Autodesk Inventor part; units mm, degrees
ref_plane "YZ Plane" through (0, 0, 0) normal (1, 0, 0) x (0, 1, 0)
ref_plane "XZ Plane" through (0, 0, 0) normal (0, 1, 0) x (-1, 0, 0)
ref_plane "XY Plane" through (0, 0, 0) normal (0, 0, 1) x (1, 0, 0)
sketch "Sketch1" plane through (0, 0, 0) normal (0, 0, 1) x (1, 0, 0)
  line L0 (55.88, 74.93) -> (55.88, 15.875)
  line L1 (55.88, 15.875) -> (43.18, 15.875)
  line L2 (43.18, 15.875) -> (42.9853, 17.3542)
  line L3 (42.9853, 17.3542) -> (42.4143, 18.7325)
  line L4 (42.4143, 18.7325) -> (41.5061, 19.9161)
  line L5 (41.5061, 19.9161) -> (40.3225, 20.8243)
  line L6 (40.3225, 20.8243) -> (38.9442, 21.3953)
  line L7 (38.9442, 21.3953) -> (37.465, 21.59)
  line L8 (37.465, 21.59) -> (19.685, 21.59)
  line L9 (19.685, 21.59) -> (18.2058, 21.3953)
  line L10 (18.2058, 21.3953) -> (16.8275, 20.8243)
  line L11 (16.8275, 20.8243) -> (15.6439, 19.9161)
  line L12 (15.6439, 19.9161) -> (14.7357, 18.7325)
  line L13 (14.7357, 18.7325) -> (14.1647, 17.3542)
  line L14 (14.1647, 17.3542) -> (13.97, 15.875)
  line L15 (13.97, 15.875) -> (1.27, 15.875)
  line L16 (1.27, 15.875) -> (1.27, 74.93)
  line L17 (1.27, 74.93) -> (1.7027, 78.217)
  line L18 (1.7027, 78.217) -> (2.9715, 81.28)
  line L19 (2.9715, 81.28) -> (4.9897, 83.9103)
  line L20 (4.9897, 83.9103) -> (7.62, 85.9285)
  line L21 (7.62, 85.9285) -> (10.683, 87.1973)
  line L22 (10.683, 87.1973) -> (13.97, 87.63)
  line L23 (13.97, 87.63) -> (43.18, 87.63)
  line L24 (43.18, 87.63) -> (46.467, 87.1973)
  line L25 (46.467, 87.1973) -> (49.53, 85.9285)
  line L26 (49.53, 85.9285) -> (52.1603, 83.9103)
  line L27 (52.1603, 83.9103) -> (54.1785, 81.28)
  line L28 (54.1785, 81.28) -> (55.4473, 78.217)
  line L29 (55.4473, 78.217) -> (55.88, 74.93)
  circle A0 centre (11.43, 81.28) radius 0.51
  circle A1 centre (13.97, 81.28) radius 0.51
  circle A2 centre (19.05, 81.28) radius 0.51
  circle A3 centre (21.59, 81.28) radius 0.51
  circle A4 centre (24.13, 81.28) radius 0.51
  circle A5 centre (26.67, 81.28) radius 0.51
extrude "untitled.brd_Outline" add sketch "Sketch1" along normal blind 1.6
properties part number "untitled.brd_Outline"
Part model, mm, in its own coordinate system. A direction names the side the tool comes from. Round coordinates to 2 decimals unless told otherwise and drop trailing zeros. Order: outer loops, then holes, each group sorted by start corner. A loop starts at its lowest first (then second) coordinate and runs counter-clockwise, first axis right, second up. Notation, with made-up numbers: (73, 43.5) -> (86, 43.5) arc R4 ccw to (86, 48.5) -> close; hole circle Ø8 at (88.5, 32.25). An arc over 180 degrees is marked (long way). Put each result on its own line as item: value.
Q1. Tool access for faces 4 (the face through (47.98, 86.57, 0.79)), 5 (the face through (39.643, 21.106, 0.789)): list every direction of +Z, -Z, +X, -X, +Y, -Y with a clear straight run to the whole face (end or side of a thin tool).
From the geometry:
face 4: +Z, -Z, +X, +Y
face 5: +Z, -Z, -Y
Q2. Wall check: line 1 (Y direction, x = 21.59, z = 0.35); line 2 (Y direction, x = 25, z = 0.35); line 3 (X direction, y = 75, z = 0.65). Give the ranges that are in metal, low to high. Write a range as [from, to].
From the geometry:
line 1: y = [21.59, 80.77], [81.79, 87.63]
line 2: y = [21.59, 87.63]
line 3: x = [1.28, 55.87]
Q3. Band-saw the part on B-B (x = 29). Give the cut face in (y, z).
From the geometry:
outline: (21.59, 0) -> (87.63, 0) -> (87.63, 1.6) -> (21.59, 1.6) -> close
Q4. Pull direction X, two halves, no side cores. Call faces 1 (the face through (55.88, 46, 1)), 2 (the face through (3.97, 82.58, 0.79)), 3 (the face through (14.454, 18.053, 0.789)): pulls with the +X half, pulls with the -X half, needs draft (parallel to the pull), parting line crosses it, or undercut.
From the geometry:
face 1: pulls with the +X half
face 2: pulls with the -X half
face 3: undercut
Q5. Pin check, flat tips, straight feed: pin 1 Ø0.8 at (x, z) = (32, 1) entering from -Y; pin 2 Ø0.9 at (x, y) = (11.43, 81.28) entering from -Z. Stop position of each tip, or through.
From the geometry:
pin 1: stops at y = 21.59
pin 2: passes through
Q6. Band-saw the part on A-A (z = 0.85). State how many separate pieces and enclosed holes the cut face has, and give its area (3 significant figures).
From the geometry:
separate pieces: 1
enclosed holes: 6
area: 3,690 mm2
